Input: part model. Units: mm. Frame: model coordinates. Face numbers are marked on the shaded views. Coordinates: 2 decimals unless noted, no trailing zeros. Loops run counter-clockwise (first coordinate to the right, second up) from the corner with the lowest first, then second, coordinate; pieces in that order, holes last. Notation, with made-up numbers: (35.25, -38.75) - (70.25, -38.75) arc R11 ccw to (70.25, -28.75) - close; hole circle Ø11 at (64, 57.25). An arc over 180 degrees is marked (long way). Use one line per item in the form item = value.
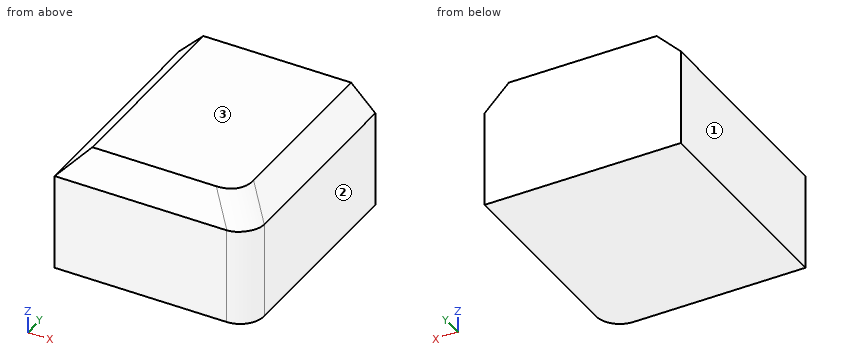
from build123d import *

# Parameters (mm, degrees)
F0_W     = 41.2199348211
F0_H     = 46.6398596764
F1_DEPTH = 25.4
F2_SIZE  = 5.08
F3_R     = 7.112
F4_R     = 5.08


with BuildPart() as f1:
    # F0 (on Top) → F1 (new body)
    with BuildSketch(Plane.XY):
        Rectangle(F0_W, F0_H)
    extrude(amount=F1_DEPTH)

    # F2
    f2_edges = [f1.edges().sort_by_distance(p)[0] for p in [
        (20.609967, 0, 25.4),
        (-20.609967, 0, 25.4),
        (0, -23.31993, 25.4),
    ]]
    chamfer(f2_edges, length=F2_SIZE)

    # F3
    f3_edges = [f1.edges().sort_by_distance(p)[0] for p in [
        (18.069967, -20.77993, 22.86),
    ]]
    fillet(f3_edges, radius=F3_R)

    # F4
    f4_edges = [f1.edges().sort_by_distance(p)[0] for p in [
        (20.609967, -23.31993, 9.486249),
    ]]
    fillet(f4_edges, radius=F4_R)


solid = f1.part
Q1. Pull-direction query (X, two-part tool) for the marked faces 1, 2 and 3; classes: pulls with the +X half, pulls with the -X half, needs draft (parallel to the pull), parting line crosses it, or undercut.
Check values:
face_1 = pulls with the -X half
face_2 = pulls with the +X half
face_3 = needs draft
Q2. Ray query, line 1 along Z through (x, y) = (-17.5, 0); line 2 along X through (y, z) = (-5, 22.5); line 3 along Z through (x, y) = (2.5, -19). Return the intervals inside material, ascending. Write a range as [from, to].
Check values:
line_1 = [0, 23.43]
line_2 = [-18.43, 18.43]
line_3 = [0, 24.64]
Q3. First-contact query: P1, Ø12, axis at x = 16, y = -0.5, coming from the -Z side. Flat tip, straight axial feed; report the tip coordinate or a pass-through.
Check values:
P1 = 0
Q4. Cut plane A-A, the plane y = 7. Return loops of the section in (x, z), then the cut area to 3 significant figures.
Check values:
outline = (-20.61, 0) - (20.61, 0) - (20.61, 20.32) - (15.53, 25.4) - (-15.53, 25.4) - (-20.61, 20.32) - close
area = 1,020 mm²
